Geometry check sheet. Reference: drawing and pictorial views, mm from the part's lowest x, y, z. A direction names the side the tool comes from. Give positions to 0.01 mm unless a question says otherwise; leave off trailing zeros. Order: outer loops, then holes, each group sorted by start corner. A loop starts at its lowest first (then second) coordinate and runs counter-clockwise, first axis right, second up. Notation, with made-up numbers: (21.5, -32) - (76.5, -32) arc R34 ccw to (76.5, 1) - close; hole circle Ø1 at (34.25, 18). An arc over 180 degrees is marked (long way). Answer in a Markdown table with one row per item.
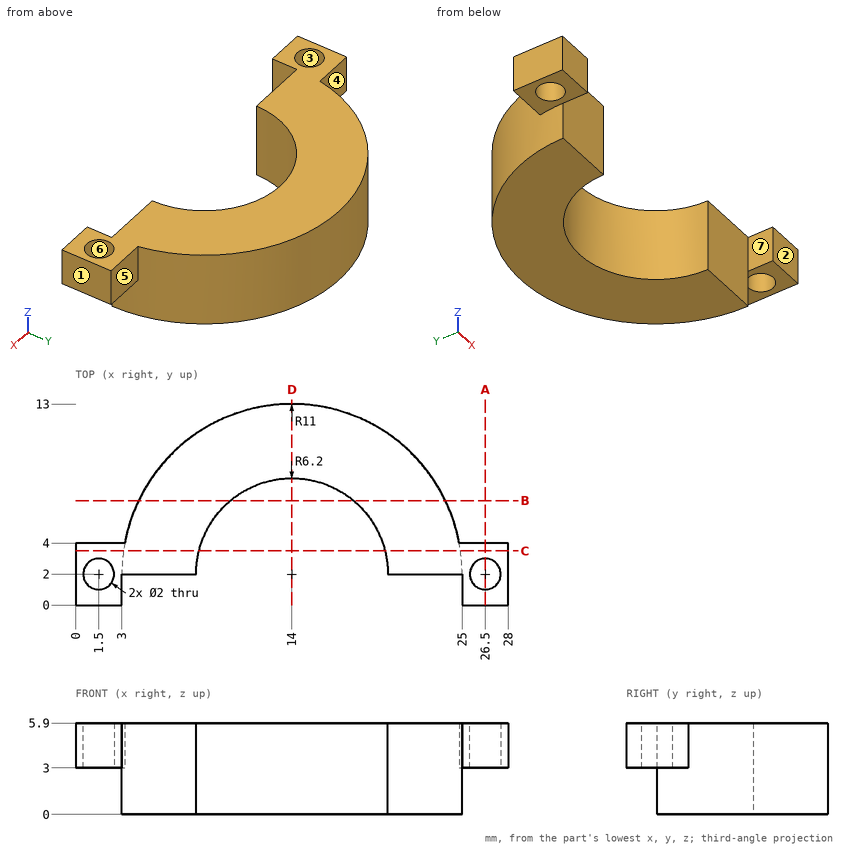
(1) Mould release check, pull along Y, two halves, no side actions. Record for the marked faces 1, 2, 3 and 4: pulls with the +Y half, pulls with the -Y half, needs draft (parallel to the pull), parting line crosses it, or undercut.
Geometry says:
| item | result |
|---|---|
| face 1 | needs draft |
| face 2 | pulls with the -Y half |
| face 3 | undercut |
| face 4 | pulls with the +Y half |
(2) Cross-section at A-A, the plane x = 26.5. Record the cut outline in (y, z), then the cut area to 3 significant figures.
Geometry says:
| item | result |
|---|---|
| outline | (0, 3) - (1, 3) - (1, 5.9) - (0, 5.9) - close; (3, 3) - (4, 3) - (4, 5.9) - (3, 5.9) - close |
| area | 5.80 mm² |
(3) Thickness scan on L1, parallel to Y at x = 26.5, z = 4.95; L2, parallel to X at y = 6.5, z = 2.35; L3, parallel to X at y = 4.25, z = 4.7. Record the ranges inside material, lowest first.
Geometry says:
| item | result |
|---|---|
| L1 | 0 to 1, 3 to 4 |
| L2 | 3.96 to 9.74, 18.26 to 24.04 |
| L3 | 3.23 to 8.22, 19.78 to 24.77 |
(4) Cross-section at B-B, the plane y = 6.75. Record the cut outline in (x, z).
Geometry says:
| item | result |
|---|---|
| outline | (4.08, 0) - (10.02, 0) - (10.02, 5.9) - (4.08, 5.9) - close; (17.98, 0) - (23.92, 0) - (23.92, 5.9) - (17.98, 5.9) - close |
(5) Cross-section at D-D, the plane x = 14. Record the cut outline in (y, z), then the cut area to 3 significant figures.
Geometry says:
| item | result |
|---|---|
| outline | (8.2, 0) - (13, 0) - (13, 5.9) - (8.2, 5.9) - close |
| area | 28.3 mm² |
(6) Gauge pin test, flat ends, axial feed: P1, Ø1.8, axis at x = 26.5, y = 2, coming from the +Z side; P2, Ø3, axis at x = 27, z = 5, coming from the +Y side; P3, Ø2, axis at y = 2, z = 1, coming from the -X side; P4, Ø3, axis at x = 16.5, z = 5, coming from the +Y side. Record the tip position at first contact, or that the pin passes through.
Geometry says:
| item | result |
|---|---|
| P1 | through |
| P2 | y = 4 |
| P3 | x = 3 |
| P4 | y = 12.95 |
(7) Cross-section at C-C, the plane y = 3.5. Record the cut outline in (x, z), then the cut area to 3 significant figures.
Geometry says:
| item | result |
|---|---|
| outline | (0, 3) - (3.1, 3) - (3.1, 0) - (7.98, 0) - (7.98, 5.9) - (0, 5.9) - close; (20.02, 0) - (24.9, 0) - (24.9, 3) - (28, 3) - (28, 5.9) - (20.02, 5.9) - close |
| area | 75.6 mm² |
(8) Access from +Z, -Z, +X, -X, +Y, -Y to the whole of each face (thin tool, end or side, straight path). Record for the marked faces 5, 6 and 7.
Geometry says:
| item | result |
|---|---|
| face 5 | +Z, -Z, +X, +Y |
| face 6 | +Z, -Z |
| face 7 | +Z, -Z, -Y |
